from build123d import *

# Parameters (mm, degrees)
SALIENTE_EXTRUIR2_DEPTH = 20
CROQUIS5_OUTSIDE_W      = 41.522
CROQUIS5_OUTSIDE_H      = 59.722
CROQUIS5_OUTSIDE_W_2    = 22.143022039
CROQUIS5_OUTSIDE_H_2    = 46.2
CORTAR_EXTRUIR1_DEPTH   = 42.444058682


with BuildPart() as part:
    # Croquis4 → Saliente-Extruir2 (new body)
    with BuildSketch(Plane(origin=(0, 0, 0), x_dir=(0, 0, -1), z_dir=(1, 0, 0))):
        with BuildLine():
            Line((0, 23.1), (28, 23.1))
            Line((28, 23.1), (28, -23.1))
            Line((28, -23.1), (0, -23.1))
            ThreePointArc((0, -23.1), (23.1, 0), (0, 23.1))
        make_face()
    extrude(amount=SALIENTE_EXTRUIR2_DEPTH)

    # Croquis5 outside → Cortar-Extruir1 (cut, through all)
    with BuildSketch(Plane(origin=(20, 0, 0), x_dir=(0, 0, -1), z_dir=(1, 0, 0))):
        with Locations((14, 0)):
            Rectangle(CROQUIS5_OUTSIDE_W, CROQUIS5_OUTSIDE_H)
        with Locations((16.92848898, 0)):
            Rectangle(CROQUIS5_OUTSIDE_W_2, CROQUIS5_OUTSIDE_H_2, mode=Mode.SUBTRACT)
    extrude(amount=-CORTAR_EXTRUIR1_DEPTH, mode=Mode.SUBTRACT)


solid = part.part
Design review of the part built by this model. Coordinates are the model's own, in mm. Round coordinates to 2 decimals unless told otherwise and drop trailing zeros. Loops run counter-clockwise (first coordinate to the right, second up) from the corner with the lowest first, then second, coordinate; pieces in that order, holes last. Notation, with made-up numbers: (14.25, 80) - (62.25, 80) arc R20 cw to (62.25, 115) - close; hole circle Ø5 at (-39.75, 30.25). An arc over 180 degrees is marked (long way). One line per question, with ' | ' between items.
1. Clearance check with a flat-ended pin moving along its axis: P1, Ø8, axis at x = 13, y = 16, coming from the +Z side. State where the tip first meets the part, or that it passes through.
Results are:
P1: stops at z = -11.56
2. For L1, parallel to Y at x = 12.5, z = -19.5; L2, parallel to Y at x = 8.25, z = -8.75; L3, parallel to Z at x = 9, y = -3, list the stretches that pass through material, from the lowest coordinate up. Write a range as [from, to].
Results are:
L1: y = [-23.1, -12.38], [12.38, 23.1] | L2: y = [-23.1, -21.38], [21.38, 23.1] | L3: z = [-28, -22.9]
3. Draft analysis for pull direction Y (two halves, no side actions). For faces 1 (the face through (10, 23.1, -17)), 2 (the face through (9.86, -0.425, -23.096)), 3 (the face through (10, -23.1, -17)), state which applies: released by +Y, released by -Y, zero draft, split by the parting line, or undercut.
Results are:
face 1: released by +Y | face 2: undercut | face 3: released by -Y
4. We need section C-C, the plane z = -19.75. State the section outline as (x, y) points.
Results are:
outline: (0, -23.1) - (20, -23.1) - (20, -11.98) - (0, -11.98) - close; (0, 11.98) - (20, 11.98) - (20, 23.1) - (0, 23.1) - close
5. We need section D-D, the plane y = -9. State the section outline as (x, z) points, and give its area (3 significant figures).
Results are:
outline: (0, -28) - (20, -28) - (20, -21.27) - (0, -21.27) - close | area: 135 mm²
6. We need section B-B, the plane x = 14.5. State the section outline as (y, z) points.
Results are:
outline: (-23.1, -28) - (23.1, -28) - (23.1, -5.86) - (22.35, -5.86) arc R23.1 cw to (-22.35, -5.86) - (-23.1, -5.86) - close
7. We need section A-A, the plane z = -8.75. State the section outline as (x, y) points.
Results are:
outline: (0, -23.1) - (20, -23.1) - (20, -21.38) - (0, -21.38) - close; (0, 21.38) - (20, 21.38) - (20, 23.1) - (0, 23.1) - close
